Answer from the drawing. Dimensions are ordinates in mm from the lowest x, y and z of the part. Give positions to 0.01 mm unless a question says otherwise; leave off trailing zeros. Loops run counter-clockwise (first coordinate to the right, second up) from the corner with the lowest first, then second, coordinate; pieces in that order, holes last. Notation, with made-up numbers: (79, -23.5) - (124, -23.5) arc R22 ccw to (124, -3.5) - close; hole circle Ø10 at (74.25, 52). An arc over 180 degrees is marked (long way). Write each question's results on one line, items separated by ' | '. Start each with the question number.
Q1. Given pin 1 (0.9 mm diameter, centred on x = 2, y = 33, fed in from +Z); pin 2 (1.5 mm diameter, centred on x = 2.5, y = 37, fed in from -Z); pin 3 (1.5 mm diameter, centred on x = 2, z = 33.5, fed in from +Y); pin 4 (5.5 mm diameter, centred on y = 33, z = 17, fed in from -X), each flat-ended and moving along its own axis, determine where each tip first touches the part or whether it passes through.
Q2. The part is cut by section A-A, the plane z = 17. Write down the section's boundary in (x, y).
Q3. The part is cut by section C-C, the plane y = 33. Write down the section's boundary in (x, z).
Q4. Find the intervals of material crossed by line 1 (Y direction, x = 1.8, z = 17); line 2 (Z direction, x = 2.5, y = 19); line 3 (Z direction, x = 2.15, y = 34), in increasing order. Write a range as from..to.
Q5. The part is cut by section D-D, the plane z = 53.2. Write down the section's boundary in (x, y), plus the area to 3 significant figures.
Q6. The part is cut by section B-B, the plane x = 0.8. Write down the section's boundary in (y, z), plus the area to 3 significant figures.
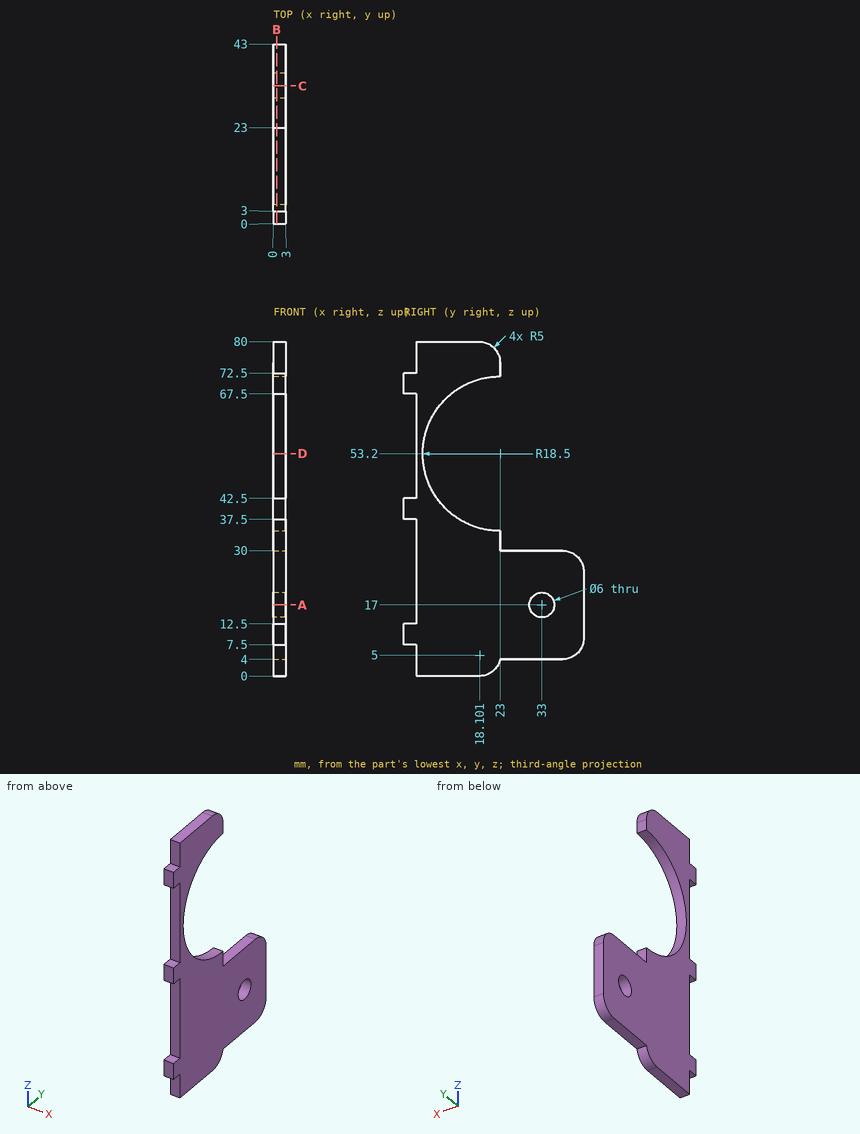
Check sheet entries:
1) pin 1: stops at z = 30 | pin 2: stops at z = 4 | pin 3: stops at y = 23 | pin 4: passes through
2) outline: (0, 3) - (3, 3) - (3, 30) - (0, 30) - close; (0, 36) - (3, 36) - (3, 43) - (0, 43) - close
3) outline: (0, 4) - (3, 4) - (3, 14) - (0, 14) - close; (0, 20) - (3, 20) - (3, 30) - (0, 30) - close
4) line 1: y = 3..30, 36..43 | line 2: z = 0.08..35.14, 71.26..79.9 | line 3: z = 4..14.17, 19.83..30
5) outline: (0, 3) - (3, 3) - (3, 4.5) - (0, 4.5) - close | area: 4.50 mm^2
6) outline: (0, 7.5) - (3, 7.5) - (3, 0) - (18.1, 0) arc R5 ccw to (23, 4) - (38, 4) arc R5 ccw to (43, 9) - (43, 25) arc R5 ccw to (38, 30) - (23, 30) - (23, 34.7) arc R18.5 cw to (23, 71.7) - (23, 75) arc R5 ccw to (18, 80) - (3, 80) - (3, 72.5) - (0, 72.5) - (0, 67.5) - (3, 67.5) - (3, 42.5) - (0, 42.5) - (0, 37.5) - (3, 37.5) - (3, 12.5) - (0, 12.5) - close; hole circle Ø6 at (33, 17) | area: 1,580 mm^2
